Source: CAD feature listing. Evaluate the final solid. Frame: model axes, mm. A direction names the side the tool comes from. Give positions to 0.01 mm unless a question says otherwise; leave off trailing zeros. Loops run counter-clockwise (first coordinate to the right, second up) from the corner with the lowest first, then second, coordinate; pieces in that order, holes last. Notation, with made-up numbers: (55, -23) -> (81, -23) arc R15 cw to (81, -1) -> close; hole circle Ø2 at (80.25, -3.5). An arc over 180 degrees is marked (long way). Return JSON: item names as keys, results as strings. Group by question number.
(1) Cut plane D-D on y = 19. Return loops of the section in (x, z) (3 decimals).
(2) Cut plane C-C on z = 6. Return loops of the section in (x, y) (3 decimals), then the cut area to 3 significant figures.
(3) Cut plane B-B on x = -0.5. Return loops of the section in (y, z) (3 decimals), then the cut area to 3 significant figures.
(4) Ray query, line 1 (X direction, y = 0.6, z = 20.32) (3 decimals); line 2 (X direction, y = 26, z = -0.5); line 3 (Y direction, x = -6, z = 4). Return the intervals inside material, ascending. Write a range as from..to.
(5) Draft query along X for faces 3 (the face through (-1, 0, 0)), 4 (the face through (-2.953, 15.79, -10.139)). Return one class per face: released by +X, released by -X, zero draft, split by the parting line, or undercut.
(6) Pin query (flat end, axial travel): pin 1 (3.5 mm diameter, centred on x = -47.625, z = 20.32, fed in from -Y); pin 2 (5 mm diameter, centred on x = 7.5, y = 19, fed in from +Z) (3 decimals); pin 3 (2 mm diameter, centred on x = -41, z = -10, fed in from +Y); pin 4 (2.5 mm diameter, centred on x = 47.625, z = -20.32, fed in from -Y). Return the tip coordinate at first contact, or that it passes through.
(7) Access query for faces 1 (the face through (-1, 1, -12)), 2 (the face through (46.126, 0.507, -20.386)). Directions: +Z, -Z, +X, -X, +Y, -Y. A direction counts if a zero-diameter tool reaches every point of the face in a straight line with its end or side. Return the directions, or none.
(8) Cut plane A-A on z = -20.32. Return loops of the section in (x, y) (3 decimals).
```python
from build123d import *

# Parameters (mm, degrees)
SCHIZZO1_W                   = 107.95
SCHIZZO1_H                   = 50.79
ESTRUSIONE_ESTRUSIONE1_DEPTH = 1
SCHIZZO2_R                   = 1.5
TAGLIO_ESTRUSIONE1_DEPTH     = 2
SCHIZZO3_R                   = 7.5
SCHIZZO3_R_2                 = 12.5
ESTRUSIONE_ESTRUSIONE2_DEPTH = 30


with BuildPart() as part:
    # Schizzo1 → Estrusione-Estrusione1 (new body)
    with BuildSketch(Plane(origin=(0, 0, 0), x_dir=(1, 0, 0), z_dir=(0, 1, 0))):
        Rectangle(SCHIZZO1_W, SCHIZZO1_H)
    extrude(amount=ESTRUSIONE_ESTRUSIONE1_DEPTH)

    # Schizzo2 → Taglio-Estrusione1 (cut, through all)
    with BuildSketch(Plane(origin=(0, 1, 0), x_dir=(1, 0, 0), z_dir=(0, 1, 0))):
        with Locations((-47.625, 20.32)):
            Circle(SCHIZZO2_R)
        with Locations((47.625, 20.32)):
            Circle(SCHIZZO2_R)
        with Locations((47.625, -20.32)):
            Circle(SCHIZZO2_R)
        with Locations((-47.625, -20.32)):
            Circle(SCHIZZO2_R)
    extrude(amount=-TAGLIO_ESTRUSIONE1_DEPTH, mode=Mode.SUBTRACT)

    # Schizzo3 → Estrusione-Estrusione2 (add)
    with BuildSketch(Plane(origin=(0, 1, 0), x_dir=(1, 0, 0), z_dir=(0, 1, 0))):
        with Locations((26.035, 3.815)):
            Circle(SCHIZZO3_R)
        with Locations((-6.985, 3.815)):
            Circle(SCHIZZO3_R)
        with Locations((9.525, -10.155)):
            Circle(SCHIZZO3_R_2)
    extrude(amount=ESTRUSIONE_ESTRUSIONE2_DEPTH)


solid = part.part
```
Answers:
{
 "1": {"outline": "circle Ø15 at (-6.985, -3.815); circle Ø25 at (9.525, 10.155); circle Ø15 at (26.035, -3.815)"},
 "2": {"outline": "(-53.975, 0) -> (53.975, 0) -> (53.975, 1) -> (21.314, 1) -> (21.314, 31) -> (-2.264, 31) -> (-2.264, 1) -> (-53.975, 1) -> close", "area": "815 mm²"},
 "3": {"outline": "(0, -25.395) -> (1, -25.395) -> (1, -7.583) -> (31, -7.583) -> (31, -0.047) -> (1, -0.047) -> (1, 2.688) -> (31, 2.688) -> (31, 17.622) -> (1, 17.622) -> (1, 25.395) -> (0, 25.395) -> close", "area": "725 mm²"},
 "4": {"line 1": "-53.975..-49.125, -46.125..46.125, 49.125..53.975", "line 2": "-13.71..-0.26, 2.99..16.06, 19.31..32.76", "line 3": "0..1"},
 "5": {"face 3": "zero draft", "face 4": "undercut"},
 "6": {"pin 1": "y = 0", "pin 2": "z = 22.655", "pin 3": "y = 1", "pin 4": "through"},
 "7": {"face 1": "+Y", "face 2": "+Y, -Y"},
 "8": {"outline": "(-53.975, 0) -> (-49.125, 0) -> (-49.125, 1) -> (-53.975, 1) -> close; (-46.125, 0) -> (46.125, 0) -> (46.125, 1) -> (-46.125, 1) -> close; (49.125, 0) -> (53.975, 0) -> (53.975, 1) -> (49.125, 1) -> close"}
}
